```python
from build123d import *

# Parameters (mm, degrees)
BOSS_EXTRUDE1_DEPTH      = 3
SKETCH2_W                = 20.0076
SKETCH2_H                = 4.999999987
BOSS_EXTRUDE2_DEPTH      = 8
BOSS_EXTRUDE3_DEPTH      = 8
SKETCH4_W                = 12.0076
SKETCH4_H                = 1.4
CUT_EXTRUDE1_DEPTH       = 27.7
M3_CLEARANCE_HOLE1_D     = 3.2
M3_CLEARANCE_HOLE1_DEPTH = 15.5
M3_CLEARANCE_HOLE1_TIP   = 0.96137699
SKETCH7_W                = 8
SKETCH7_H                = 0.4
CUT_EXTRUDE2_DEPTH       = 28.5
BOSS_EXTRUDE4_DEPTH      = 4.6
BOSS_EXTRUDE5_DEPTH      = 3.647111
SKETCH10_W               = 25.759770256
SKETCH10_H               = 7.605956873
CUT_EXTRUDE3_DEPTH       = 15


with BuildPart() as part:
    # Sketch1 → Boss-Extrude1 (new body)
    with BuildSketch(Plane.XY):
        Polygon((24.618539046, -84.902707764), (24.618539046, -85.849818272), (20.618539046, -85.849818272), (20.618539046, -73.202707764), (40.626139046, -73.202707764), (40.626139046, -85.849818272), (36.626139046, -85.849818272), (36.626139046, -84.902707764), align=None)
    extrude(amount=BOSS_EXTRUDE1_DEPTH)

    # Sketch2 → Boss-Extrude2 (add)
    with BuildSketch(Plane(origin=(0, 0, 0), x_dir=(-1, 0, 0), z_dir=(0, 0, -1))):
        with Locations((-30.622339046, -75.702707758)):
            Rectangle(SKETCH2_W, SKETCH2_H)
    extrude(amount=BOSS_EXTRUDE2_DEPTH)

    # Sketch3 → Boss-Extrude3 (add)
    with BuildSketch(Plane(origin=(0, 0, 0), x_dir=(-1, 0, 0), z_dir=(0, 0, -1))):
        Polygon((-40.626139046, -82.202707751), (-40.626139046, -85.849818272), (-36.626139046, -85.849818272), (-36.626139046, -84.902707764), (-24.618539046, -84.902707764), (-24.618539046, -85.849818272), (-20.618539046, -85.849818272), (-20.618539046, -82.202707751), align=None)
    extrude(amount=BOSS_EXTRUDE3_DEPTH)

    # Sketch4 → Cut-Extrude1 (cut)
    with BuildSketch(Plane.XY.offset(3)):
        with Locations((30.622339046, -73.902707764)):
            Rectangle(SKETCH4_W, SKETCH4_H)
    extrude(amount=-CUT_EXTRUDE1_DEPTH, mode=Mode.SUBTRACT)

    # M3 Clearance Hole1
    with Locations(Plane(origin=(0, -73.202707764, 0), x_dir=(1, 0, 0), z_dir=(0, 1, 0))):
        with Locations((22.618539046, 6), (38.626139046, 6)):
            Hole(M3_CLEARANCE_HOLE1_D / 2, depth=M3_CLEARANCE_HOLE1_DEPTH)
            with Locations((0, 0, -(M3_CLEARANCE_HOLE1_DEPTH + M3_CLEARANCE_HOLE1_TIP / 2))):  # 118° drill point
                Cone(0, M3_CLEARANCE_HOLE1_D / 2, M3_CLEARANCE_HOLE1_TIP, mode=Mode.SUBTRACT)

    # Sketch7 → Cut-Extrude2 (cut)
    with BuildSketch(Plane(origin=(40.626139046, 0, 0), x_dir=(0, 0, -1), z_dir=(1, 0, 0))):
        with Locations((4, -78.002707751)):
            Rectangle(SKETCH7_W, SKETCH7_H)
    extrude(amount=-CUT_EXTRUDE2_DEPTH, mode=Mode.SUBTRACT)

    # Sketch8 → Boss-Extrude4 (add)
    with BuildSketch(Plane(origin=(0, -73.202707764, 0), x_dir=(1, 0, 0), z_dir=(0, 1, 0))):
        with BuildLine():
            ThreePointArc((24.618539046, 8), (22.618539046, 8.828427125), (20.618539046, 8))
            Line((20.618539046, 8), (24.618539046, 8))
        make_face()
        with BuildLine():
            ThreePointArc((20.618539046, 8), (19.790111921, 6), (20.618539046, 4))
            Line((20.618539046, 4), (20.618539046, 8))
        make_face()
        with BuildLine():
            Line((36.626139046, 8), (40.626139046, 8))
            ThreePointArc((40.626139046, 8), (38.626139046, 8.828427125), (36.626139046, 8))
        make_face()
        with BuildLine():
            ThreePointArc((40.626139046, 4), (41.45456617, 6), (40.626139046, 8))
            Line((40.626139046, 8), (40.626139046, 4))
        make_face()
    extrude(amount=-BOSS_EXTRUDE4_DEPTH)

    # Sketch9 → Boss-Extrude5 (add)
    with BuildSketch(Plane.XZ.offset(85.849818272)):
        with BuildLine():
            Line((20.618539046, -8), (20.618539046, -4))
            ThreePointArc((20.618539046, -4), (19.790111921, -6), (20.618539046, -8))
        make_face()
        with BuildLine():
            Line((24.618539046, -8), (20.618539046, -8))
            ThreePointArc((20.618539046, -8), (22.618539046, -8.828427125), (24.618539046, -8))
        make_face()
        with BuildLine():
            Line((40.626139046, -8), (36.626139046, -8))
            ThreePointArc((36.626139046, -8), (38.626139046, -8.828427125), (40.626139046, -8))
        make_face()
        with BuildLine():
            Line((40.626139046, -4), (40.626139046, -8))
            ThreePointArc((40.626139046, -8), (41.45456617, -6), (40.626139046, -4))
        make_face()
    extrude(amount=-BOSS_EXTRUDE5_DEPTH)

    # Sketch10 → Cut-Extrude3 (cut)
    with BuildSketch(Plane.XY.offset(3)):
        with Locations((29.890783296, -73.999729313)):
            Rectangle(SKETCH10_W, SKETCH10_H)
    extrude(amount=-CUT_EXTRUDE3_DEPTH, mode=Mode.SUBTRACT)


solid = part.part
```
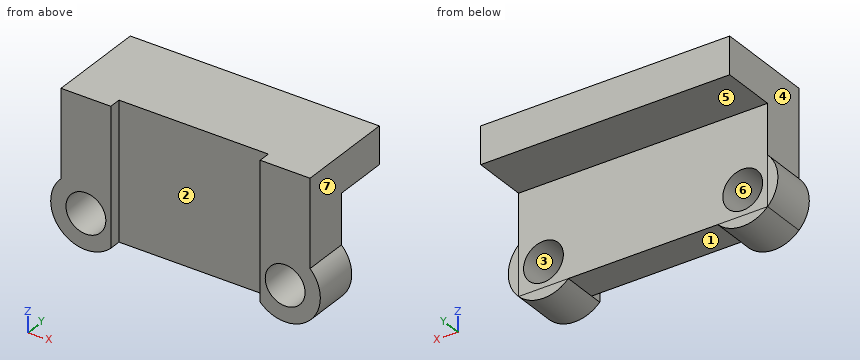
Can you work these out from the model? Positions are in its coordinate system, mm. Face numbers are marked on the shaded views. A direction names the side the tool comes from. Coordinates: 2 decimals unless noted, no trailing zeros. Loops run counter-clockwise (first coordinate to the right, second up) from the corner with the lowest first, then second, coordinate; pieces in that order, holes last.
1) Which directions (+Z, -Z, +X, -X, +Y, -Y) give clear straight access to the entire face, cutting with the end or side of a thin tool? Please do the marked faces 1, 2, 3 and 4.
2) For pin 1 (6 mm diameter, centred on x = 34.5, z = -4, fed in from +Y); pin 2 (3.5 mm diameter, centred on y = -81.5, z = -2, fed in from -X); pin 3 (1.3 mm diameter, centred on x = 27.5, y = -79.5, fed in from -Z), each with a flat end and sliding along its axis, tell me the tip position at first contact or that it passes through.
3) Imagine slicing it at A-A on z = -6. List the corners of the cut face in (x, y) for me.
4) I need wall thicknesses on probe 1 along X at (y, z) = (-83.2, -6); probe 2 along Z at (x, y) = (25, -82.75); probe 3 along Y at (x, z) = (23.25, -8). Which ranges of each line are inside material? Lowest first, please.
5) Imagine slicing it at D-D on z = -1.75. List the corners of the cut face in (x, y) for me, plus the area to 3 significant figures.
6) Thinking about a two-plate mould opening in X: for the marked faces 5, 6 and 7, which applies, pulls with the +X half, pulls with the -X half, needs draft (parallel to the pull), parting line crosses it, or undercut?
7) Imagine slicing it at B-B on y = -83.5. List the corners of the cut face in (x, z) for me, plus the area to 3 significant figures.
8) Imagine slicing it at C-C on x = 38.25. List the corners of the cut face in (y, z) for me, plus the area to 3 significant figures.
Completed:
1. face 1: -Z, +Y, -Y
1. face 2: +Z, -Z, -Y
1. face 3: +Y, -Y
1. face 4: +Z, -X, +Y, -Y
2. pin 1: stops at y = -82.2
2. pin 2: stops at x = 20.62
2. pin 3: stops at z = 0
3. outline: (19.79, -85.85) - (21.02, -85.85) - (21.02, -82.2) - (19.79, -82.2) - close; (24.22, -85.85) - (24.62, -85.85) - (24.62, -84.9) - (36.63, -84.9) - (36.63, -85.85) - (37.03, -85.85) - (37.03, -82.2) - (24.22, -82.2) - close; (40.23, -85.85) - (41.45, -85.85) - (41.45, -82.2) - (40.23, -82.2) - close
4. probe 1: x = 19.79 to 21.02, 24.22 to 37.03, 40.23 to 41.45
4. probe 2: z = -8 to 3
4. probe 3: y = -85.85 to -82.2
5. outline: (20.62, -85.85) - (24.62, -85.85) - (24.62, -84.9) - (36.63, -84.9) - (36.63, -85.85) - (40.63, -85.85) - (40.63, -82.2) - (20.62, -82.2) - close
5. area: 61.6 mm2
6. face 5: needs draft
6. face 6: undercut
6. face 7: pulls with the +X half
7. outline: (20.62, -4) arc R2.83 ccw to (24.62, -8) - (36.63, -8) arc R2.83 ccw to (40.63, -4) - (40.63, 3) - (20.62, 3) - close; hole circle Ø3.2 at (22.62, -6); hole circle Ø3.2 at (38.63, -6)
7. area: 213 mm2
8. outline: (-85.85, -8.8) - (-82.2, -8.8) - (-82.2, -7.56) - (-85.85, -7.56) - close; (-85.85, -4.44) - (-82.2, -4.44) - (-82.2, 0) - (-77.8, 0) - (-77.8, 3) - (-85.85, 3) - close
8. area: 44.9 mm2
